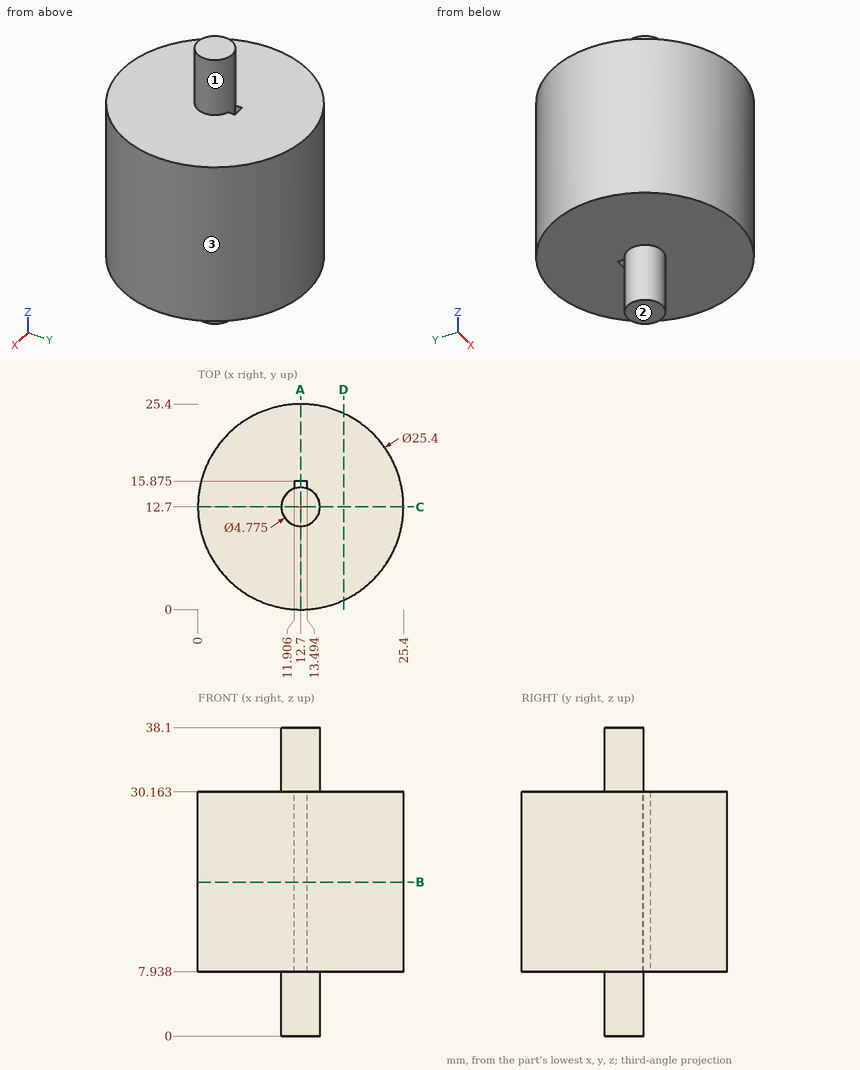
Verification items for this drawing (mm, ordinates from the low corner). Coordinates: 2 decimals unless noted, no trailing zeros. Loops run counter-clockwise (first coordinate to the right, second up) from the corner with the lowest first, then second, coordinate; pieces in that order, holes last. Notation, with made-up numbers: (-0.5, 27.25) -> (39.5, 27.25) arc R19 cw to (39.5, 52.25) -> close; hole circle Ø10 at (23.5, -14). An arc over 180 degrees is marked (long way). Put each result on its own line as item: value.
1. Section check A-A, the plane x = 12.7. Record the boundary of the cut face in (y, z) (1 decimal).
Result set:
outline: (0, 7.9) -> (10.3, 7.9) -> (10.3, 0) -> (15.1, 0) -> (15.1, 38.1) -> (10.3, 38.1) -> (10.3, 30.2) -> (0, 30.2) -> close; (15.9, 7.9) -> (25.4, 7.9) -> (25.4, 30.2) -> (15.9, 30.2) -> close
2. Section check B-B, the plane z = 19. Record the boundary of the cut face in (x, y) (1 decimal).
Result set:
outline: circle Ø25.4 at (12.7, 12.7); hole (11.9, 15) arc R2.4 cw to (13.5, 15) -> (13.5, 15.9) -> (11.9, 15.9) -> close
3. Section check D-D, the plane x = 18. Record the boundary of the cut face in (y, z).
Result set:
outline: (1.16, 7.94) -> (24.24, 7.94) -> (24.24, 30.16) -> (1.16, 30.16) -> close
4. Section check C-C, the plane y = 12.7. Record the boundary of the cut face in (x, z).
Result set:
outline: (0, 7.94) -> (10.31, 7.94) -> (10.31, 0) -> (15.09, 0) -> (15.09, 7.94) -> (25.4, 7.94) -> (25.4, 30.16) -> (15.09, 30.16) -> (15.09, 38.1) -> (10.31, 38.1) -> (10.31, 30.16) -> (0, 30.16) -> close
5. Gauge pin test, flat ends, axial feed: P1, Ø2, axis at x = 3.5, z = 17.5, coming from the -Y side; P2, Ø3, axis at x = 20, z = 8.5, coming from the +Y side; P3, Ø1, axis at y = 15.5, z = 15.5, coming from the +X side. Record the tip position at first contact, or that the pin passes through.
Result set:
P1: stops at y = 3
P2: stops at y = 24
P3: stops at x = 25.19
6. Thickness scan on line 1 (Z direction, x = 18, y = 8.5); line 2 (X direction, y = 18.5, z = 27.5); line 3 (Y direction, x = 16.25, z = 18) (1 decimal). Record the ranges inside material, lowest first.
Result set:
line 1: z = 7.94 to 30.16
line 2: x = 1.4 to 24
line 3: y = 0.5 to 24.9
7. Mould release check, pull along Y, two halves, no side actions. Record for the marked faces 1, 2 and 3: pulls with the +Y half, pulls with the -Y half, needs draft (parallel to the pull), parting line crosses it, or undercut.
Result set:
face 1: undercut
face 2: needs draft
face 3: parting line crosses it
